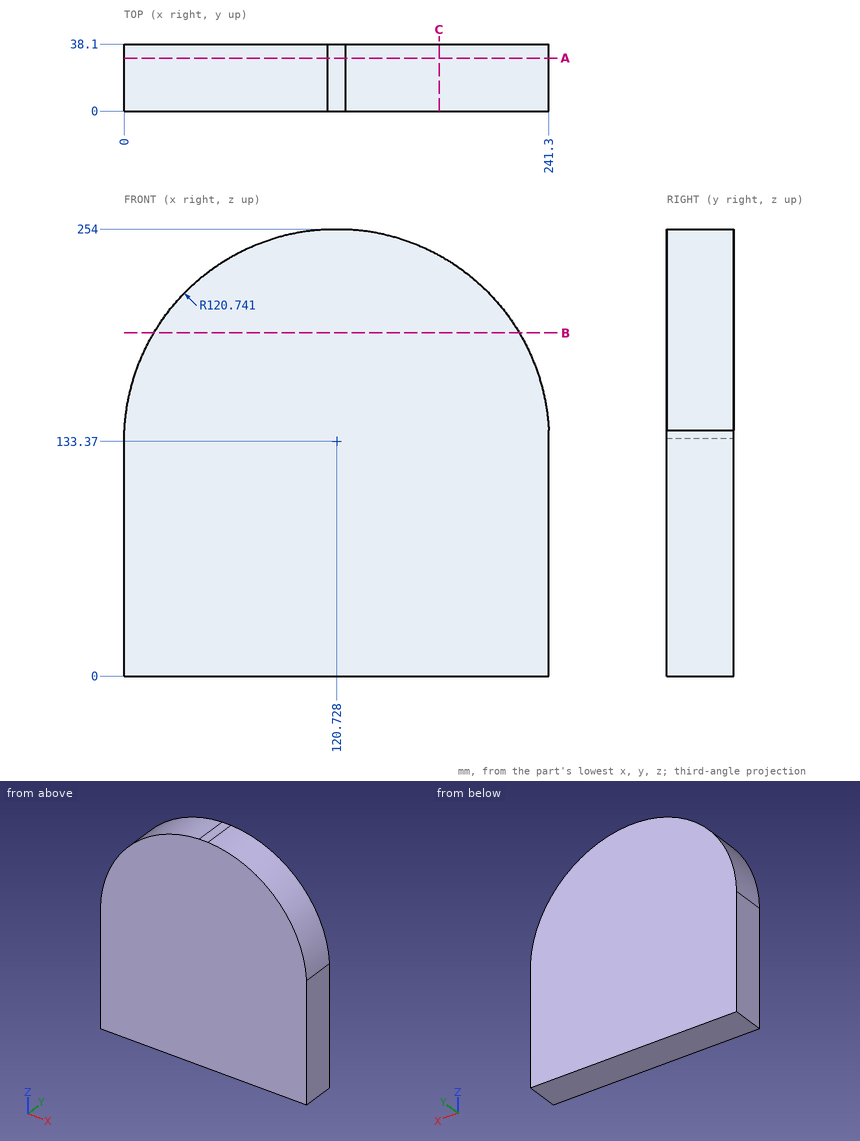
Print and shaded views of the part. All mm, measured from the part's lowest x, y and z. Give positions to 0.01 mm unless a question says otherwise; leave off trailing zeros. Loops run counter-clockwise (first coordinate to the right, second up) from the corner with the lowest first, then second, coordinate; pieces in that order, holes last. Notation, with made-up numbers: (88, 3.5) -> (119, 3.5) arc R26 ccw to (119, 23.5) -> close; hole circle Ø11 at (39.5, -10.75). An arc over 180 degrees is marked (long way). Use a Markdown table: item, result.
1. Slice it at C-C (x = 179). List the corners of the cut face in (y, z).
Check result:
| item | result |
|---|---|
| outline | (0, 0) -> (38.1, 0) -> (38.1, 239.12) -> (0, 239.12) -> close |
2. Wall check: L1, parallel to Z at x = 20, y = 13.5 (1 decimal); L2, parallel to X at y = 8, z = 215 (1 decimal); L3, parallel to Z at x = 113, y = 18. Give the ranges that are in metal, low to high. Write a range as [from, to].
Check result:
| item | result |
|---|---|
| L1 | z = [0, 199.9] |
| L2 | x = [31.8, 209.7] |
| L3 | z = [0, 253.86] |
3. Slice it at B-B (z = 195). List the corners of the cut face in (x, y) (1 decimal), plus the area to 3 significant figures.
Check result:
| item | result |
|---|---|
| outline | (16.9, 0) -> (224.6, 0) -> (224.6, 38.1) -> (16.9, 38.1) -> close |
| area | 7,910 mm^2 |
4. Slice it at A-A (y = 30). List the corners of the cut face in (x, z).
Check result:
| item | result |
|---|---|
| outline | (0, 0) -> (241.3, 0) -> (241.3, 139.74) arc R120.74 ccw to (125.89, 254) -> (115.56, 254) arc R120.74 ccw to (0, 135.13) -> close |
5. Flat gauge pins, fed straight in: pin 1 (10 mm diameter, centred on y = 29, z = 154.5, fed in from +X); pin 2 (12 mm diameter, centred on x = 58.5, y = 23, fed in from +Z); pin 3 (6 mm diameter, centred on y = 18.5, z = 182, fed in from -X). Where does each tip first touch, or does it go through?
Check result:
| item | result |
|---|---|
| pin 1 | stops at x = 240.39 |
| pin 2 | stops at z = 240.22 |
| pin 3 | stops at x = 8.94 |
